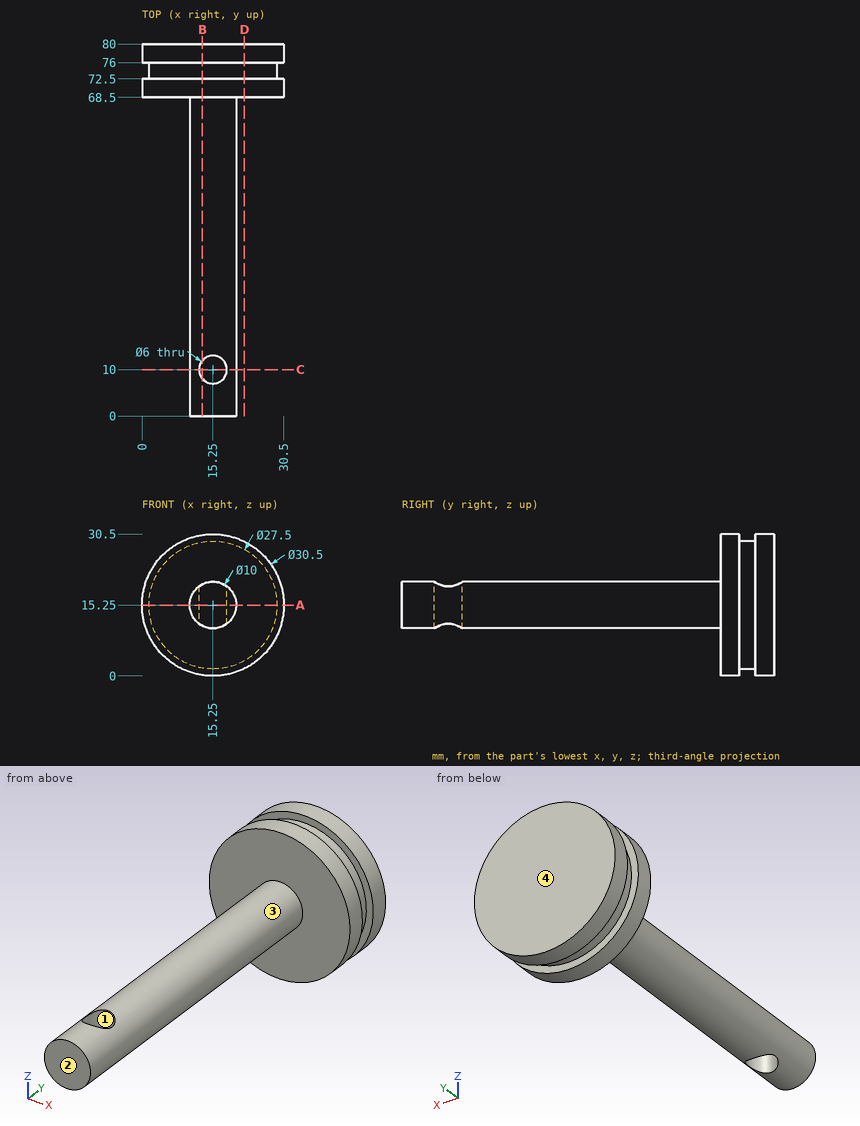
The drawing under review shows one solid part. Ordinate dimensions are in mm from its lowest x, y, z. Round coordinates to 2 decimals unless told otherwise and drop trailing zeros. Order: outer loops, then holes, each group sorted by start corner. A loop starts at its lowest first (then second) coordinate and runs counter-clockwise, first axis right, second up. Notation, with made-up numbers: (61, 19) - (71, 19) arc R32 ccw to (71, 56) - close; hole circle Ø5 at (88.5, 55.25). An arc over 180 degrees is marked (long way). Return JSON: item names as keys, results as strings.
Q1. Consider section B-B on x = 13. Write out the cut boundary in (y, z).
Computed values:
{"outline": "(0, 10.78) - (8.02, 10.78) - (8.02, 19.72) - (0, 19.72) - close; (11.98, 10.78) - (68.5, 10.78) - (68.5, 0.17) - (72.5, 0.17) - (72.5, 1.69) - (76, 1.69) - (76, 0.17) - (80, 0.17) - (80, 30.33) - (76, 30.33) - (76, 28.81) - (72.5, 28.81) - (72.5, 30.33) - (68.5, 30.33) - (68.5, 19.72) - (11.98, 19.72) - close"}
Q2. The part is to be moulded in two halves that separate along Y. For the marked faces 1, 2, 3 and 4, say which applies: pulls with the +Y half, pulls with the -Y half, needs draft (parallel to the pull), parting line crosses it, or undercut.
Computed values:
{"face 1": "undercut", "face 2": "pulls with the -Y half", "face 3": "needs draft", "face 4": "pulls with the +Y half"}
Q3. For pin 1 Ø3 at (y, z) = (23.5, 10) entering from +X; pin 2 Ø5 at (x, z) = (9, 3.5) entering from -Y; pin 3 Ø6 at (x, y) = (21.5, 67.5) entering from -Z; pin 4 Ø3 at (y, z) = (65, 8) entering from -X, all flat-tipped, find the tip position at first contact; note any pin that passes through.
Computed values:
{"pin 1": "stops at x = 18.56", "pin 2": "stops at y = 68.5", "pin 3": "stops at z = 0.39", "pin 4": "passes through"}
Q4. Consider section D-D on x = 22. Write out the cut boundary in (y, z).
Computed values:
{"outline": "(68.5, 1.58) - (72.5, 1.58) - (72.5, 3.27) - (76, 3.27) - (76, 1.58) - (80, 1.58) - (80, 28.92) - (76, 28.92) - (76, 27.23) - (72.5, 27.23) - (72.5, 28.92) - (68.5, 28.92) - close"}
Q5. Consider section C-C on y = 10. Write out the cut boundary in (x, z), plus the area to 3 significant figures.
Computed values:
{"outline": "(12.25, 11.25) - (12.25, 19.25) arc R5 ccw to start; (18.25, 11.25) arc R5 ccw to (18.25, 19.25) - close", "area": "22.4 mm2"}
Q6. Consider section A-A on z = 15.25. Write out the cut boundary in (x, y), plus the area to 3 significant figures.
Computed values:
{"outline": "(0, 68.5) - (10.25, 68.5) - (10.25, 0) - (20.25, 0) - (20.25, 68.5) - (30.5, 68.5) - (30.5, 72.5) - (29, 72.5) - (29, 76) - (30.5, 76) - (30.5, 80) - (0, 80) - (0, 76) - (1.5, 76) - (1.5, 72.5) - (0, 72.5) - close; hole circle Ø6 at (15.25, 10)", "area": "997 mm2"}
Q7. Wall thickness on L1, parallel to Y at x = 29.5, z = 14.5; L2, parallel to Y at x = 15, z = 16; L3, parallel to Y at x = 8, z = 24.5: over which ranges is each line inside the solid? List them lowest first. Write a range as [from, to].
Computed values:
{"L1": "y = [68.5, 72.5], [76, 80]", "L2": "y = [0, 7.01], [12.99, 80]", "L3": "y = [68.5, 80]"}
